```python
from build123d import *

# Parameters (mm, degrees)
SKIZZE1_R                       = 15
SKIZZE1_R_2                     = 7
SKIZZE1_R_3                     = 1.65
AUFSATZ_LINEAR_AUSTRAGEN1_DEPTH = 36.5
SKIZZE2_R                       = 2.9
SCHNITT_LINEAR_AUSTRAGEN1_DEPTH = 24.5
SKIZZE3_R                       = 2.5
SCHNITT_LINEAR_AUSTRAGEN2_DEPTH = 5


with BuildPart() as part:
    # Skizze1 → Aufsatz-Linear austragen1 (new body)
    with BuildSketch(Plane.XY):
        Circle(SKIZZE1_R)
        Circle(SKIZZE1_R_2, mode=Mode.SUBTRACT)
        with Locations((-11, 0)):
            Circle(SKIZZE1_R_3, mode=Mode.SUBTRACT)
        with Locations((0, 11)):
            Circle(SKIZZE1_R_3, mode=Mode.SUBTRACT)
        with Locations((11, 0)):
            Circle(SKIZZE1_R_3, mode=Mode.SUBTRACT)
        with Locations((0, -11)):
            Circle(SKIZZE1_R_3, mode=Mode.SUBTRACT)
    extrude(amount=AUFSATZ_LINEAR_AUSTRAGEN1_DEPTH)

    # Skizze2 → Schnitt-Linear austragen1 (cut)
    with BuildSketch(Plane.XY.offset(36.5)):
        with Locations((-11, 0)):
            Circle(SKIZZE2_R)
        with Locations((0, 11)):
            Circle(SKIZZE2_R)
        with Locations((11, 0)):
            Circle(SKIZZE2_R)
        with Locations((0, -11)):
            Circle(SKIZZE2_R)
    extrude(amount=-SCHNITT_LINEAR_AUSTRAGEN1_DEPTH, mode=Mode.SUBTRACT)

    # Skizze3 → Schnitt-Linear austragen2 (cut)
    with BuildSketch(Plane.XY.offset(36.5)):
        with Locations((-7.778174593, 7.778174593)):
            Circle(SKIZZE3_R)
        with Locations((7.778174593, 7.778174593)):
            Circle(SKIZZE3_R)
        with Locations((7.778174593, -7.778174593)):
            Circle(SKIZZE3_R)
        with Locations((-7.778174593, -7.778174593)):
            Circle(SKIZZE3_R)
    extrude(amount=-SCHNITT_LINEAR_AUSTRAGEN2_DEPTH, mode=Mode.SUBTRACT)


solid = part.part
```
Build history of the part. All positions in model axes, mm. A direction names the side the tool comes from. Round coordinates to 2 decimals unless told otherwise and drop trailing zeros. Write each loop counter-clockwise with the first axis right and the second up, starting at its lowest first coordinate (ties: lowest second). Pieces come first, ordered by that corner, then holes. Notation, with made-up numbers: (54, 28) -> (76, 28) arc R23 cw to (76, 52) -> close; hole circle Ø4 at (29, -15.5). An arc over 180 degrees is marked (long way). Put each result on its own line as item: value.
Item 1: Slice it at C-C, the plane z = 10. Give the cut face in (x, y), plus the area to 3 significant figures.
Here are the results:
outline: circle Ø30 at (0, 0); hole circle Ø3.3 at (-11, 0); hole circle Ø14 at (0, 0); hole circle Ø3.3 at (0, -11); hole circle Ø3.3 at (0, 11); hole circle Ø3.3 at (11, 0)
area: 519 mm^2
Item 2: Slice it at A-A, the plane x = 0. Give the cut face in (y, z).
Here are the results:
outline: (-15, 0) -> (-12.65, 0) -> (-12.65, 12) -> (-13.9, 12) -> (-13.9, 36.5) -> (-15, 36.5) -> close; (-9.35, 0) -> (-7, 0) -> (-7, 36.5) -> (-8.1, 36.5) -> (-8.1, 12) -> (-9.35, 12) -> close; (7, 0) -> (9.35, 0) -> (9.35, 12) -> (8.1, 12) -> (8.1, 36.5) -> (7, 36.5) -> close; (12.65, 0) -> (15, 0) -> (15, 36.5) -> (13.9, 36.5) -> (13.9, 12) -> (12.65, 12) -> close
Item 3: Slice it at D-D, the plane x = 11. Give the cut face in (y, z).
Here are the results:
outline: (-10.2, 0) -> (-1.65, 0) -> (-1.65, 12) -> (-2.9, 12) -> (-2.9, 36.5) -> (-10.2, 36.5) -> close; (1.65, 0) -> (10.2, 0) -> (10.2, 36.5) -> (2.9, 36.5) -> (2.9, 12) -> (1.65, 12) -> close
Item 4: Two-plate mould, pull along X, no slides. Class faces 1 (the face through (-14.985, 0.66, 17.994)), 2 (the face through (6.466, -2.681, 17.994)), 3 (the face through (6.5, -3.1, 0)), 4 (the face through (-8, 8, 31.5)): pulls with the +X half, pulls with the -X half, needs draft (parallel to the pull), parting line crosses it, or undercut.
Here are the results:
face 1: parting line crosses it
face 2: undercut
face 3: needs draft
face 4: undercut
Item 5: Flat gauge pins, fed straight in: P1, Ø1.5, axis at x = 8.5, z = 20.5, coming from the +Y side; P2, Ø2, axis at x = 11, y = 0, coming from the +Z side; P3, Ø2, axis at x = -9.5, z = 30, coming from the +Y side; P4, Ø3, axis at x = -7.78, y = -7.78, coming from the +Z side. Where does each tip first touch, or does it go through?
Here are the results:
P1: stops at y = 12.84
P2: passes through
P3: stops at y = 12.36
P4: stops at z = 31.5
Item 6: Wall check: probe 1 along Y at (x, z) = (0, 10); probe 2 along Y at (x, z) = (0, 19); probe 3 along X at (y, z) = (-0.75, 23). Give the ranges that are in metal, low to high. Write a range as from..to.
Here are the results:
probe 1: y = -15..-12.65, -9.35..-7, 7..9.35, 12.65..15
probe 2: y = -15..-13.9, -8.1..-7, 7..8.1, 13.9..15
probe 3: x = -14.98..-13.8, -8.2..-6.96, 6.96..8.2, 13.8..14.98
Item 7: Tool access for faces 5 (the face through (-0.4, -12.6, 5.9)), 6 (the face through (0, 9, 12)): list every direction of +Z, -Z, +X, -X, +Y, -Y with a clear straight run to the whole face (end or side of a thin tool).
Here are the results:
face 5: +Z, -Z
face 6: +Z
